```python
from build123d import *

# Parameters (mm, degrees)
SKETCH_1_W                  = 56
SKETCH_1_H                  = 90
SKETCH_1_R                  = 1.6
EXTRUDE_1_DEPTH             = 3
SKETCH_2_R                  = 18.5
SKETCH_2_R_2                = 1.6
CUT_EXTRUDE_1_DEPTH         = 54.08483776
FILLET_1_R                  = 2
CUT_EXTRUDE_2_DEPTH         = 54.08483776
FILLET_2_R                  = 2
HOLE_WIZARD_M3_1_AT_2_COUNT = 2
HOLE_WIZARD_M3_1_AT_2_PITCH = 63.694583757
HOLE_WIZARD_M3_1_AT_3_COUNT = 2
HOLE_WIZARD_M3_1_AT_3_PITCH = 63.694583757


with BuildPart() as part:
    # 草图1 → 凸台-拉伸1 (new body)
    with BuildSketch(Plane.XY):
        Rectangle(SKETCH_1_W, SKETCH_1_H)
        with Locations((10, 42)):
            Circle(SKETCH_1_R, mode=Mode.SUBTRACT)
        with Locations(Location((-10, 42, 0), (0, 0, 180))):
            Circle(SKETCH_1_R, mode=Mode.SUBTRACT)
    extrude(amount=EXTRUDE_1_DEPTH)

    # 草图2 → 切除-拉伸1 (cut, through all)
    with BuildSketch(Plane.XY.offset(3)):
        with Locations((0, -17)):
            Circle(SKETCH_2_R)
        with Locations((0, 18)):
            Circle(SKETCH_2_R_2)
        with Locations((24, -41)):
            Circle(SKETCH_2_R_2)
        with Locations(Location((-24, -41, 0), (0, 0, 180))):
            Circle(SKETCH_2_R_2)
    extrude(amount=-CUT_EXTRUDE_1_DEPTH, mode=Mode.SUBTRACT)

    # 圆角1
    fillet_1_edges = [part.edges().sort_by_distance(p)[0] for p in [
        (28, -45, 1.5),
        (-28, -45, 1.5),
        (-28, 45, 1.5),
        (28, 45, 1.5),
    ]]
    fillet(fillet_1_edges, radius=FILLET_1_R)

    # 草图3 → 切除-拉伸2 (cut, through all)
    with BuildSketch(Plane.XY.offset(3)):
        Polygon((-23.345028529, 37.432122744), (-4.29507275, 37.432122744), (-4.29507275, 6.166928146), (-23.345028529, -1.831144891), align=None)
        Polygon((4.29507275, 6.166928146), (23.345028529, -1.831144891), (23.345028529, 37.432122744), (4.29507275, 37.432122744), align=None)
        Polygon((-21.449213, -21.510239836), (-24.998316916, -30.185827186), (-17.308591765, -43.00203577), (-5.576831599, -43.00203577), (-16.421315786, -33.044827562), align=None)
        Polygon((21.449213, -21.510239836), (24.998316916, -30.185827186), (17.308591765, -43.00203577), (5.576831599, -43.00203577), (16.421315786, -33.044827562), align=None)
    extrude(amount=-CUT_EXTRUDE_2_DEPTH, mode=Mode.SUBTRACT)

    # 圆角2
    fillet_2_edges = [part.edges().sort_by_distance(p)[0] for p in [
        (-5.576831599, -43.00203577, 1.5),
        (-17.308591765, -43.00203577, 1.5),
        (-24.998316916, -30.185827186, 1.5),
        (-21.449213, -21.510239836, 1.5),
        (-16.421315786, -33.044827562, 1.5),
        (-23.345028529, -1.831144891, 1.5),
        (-23.345028529, 37.432122744, 1.5),
        (-4.29507275, 37.432122744, 1.5),
        (-4.29507275, 6.166928146, 1.5),
        (4.29507275, 6.166928146, 1.5),
        (4.29507275, 37.432122744, 1.5),
        (23.345028529, 37.432122744, 1.5),
        (23.345028529, -1.831144891, 1.5),
        (16.421315786, -33.044827562, 1.5),
        (21.449213, -21.510239836, 1.5),
        (24.998316916, -30.185827186, 1.5),
        (17.308591765, -43.00203577, 1.5),
        (5.576831599, -43.00203577, 1.5),
    ]]
    fillet(fillet_2_edges, radius=FILLET_2_R)

    # 草图5 → M3 十字槽半沉头木螺钉的锥形沉头孔1 (revolve, cut)
    with BuildSketch(Plane(origin=(0, 18, 0), x_dir=(0, 1, 0), z_dir=(1, 0, 0))):
        Polygon((0, 0), (0, 3), (1.8, 3), (1.8, 1.5), (3.3, 0), align=None)
    hole_wizard_m3_1 = revolve(axis=Axis((0, 18, -6.35), (0, 0, 1)), mode=Mode.SUBTRACT)

    # M3 十字槽半沉头木螺钉的锥形沉头孔1 at 2: M3 十字槽半沉头木螺钉的锥形沉头孔1 ×2
    with Locations(*[Vector(-0.3767981292019326, -0.9262954009547514, 0) * (i * HOLE_WIZARD_M3_1_AT_2_PITCH) for i in range(1, HOLE_WIZARD_M3_1_AT_2_COUNT)]):
        add(hole_wizard_m3_1, mode=Mode.SUBTRACT)

    # M3 十字槽半沉头木螺钉的锥形沉头孔1 at 3: M3 十字槽半沉头木螺钉的锥形沉头孔1 ×2
    with Locations(*[Vector(0.3767981292019329, -0.9262954009547514, 0) * (i * HOLE_WIZARD_M3_1_AT_3_PITCH) for i in range(1, HOLE_WIZARD_M3_1_AT_3_COUNT)]):
        add(hole_wizard_m3_1, mode=Mode.SUBTRACT)


solid = part.part
```
Model file for the job. Use its own axes, mm. A direction names the side the tool comes from. Give positions to 0.01 mm unless a question says otherwise; leave off trailing zeros. Loops run counter-clockwise (first coordinate to the right, second up) from the corner with the lowest first, then second, coordinate; pieces in that order, holes last. Notation, with made-up numbers: (20, 49.25) - (47, 49.25) arc R27 ccw to (47, 86.25) - close; hole circle Ø9 at (43.25, 62). An arc over 180 degrees is marked (long way). One line per item, written item: value. Start each with the question number.
1. Slice it at A-A (y = -17). List the corners of the cut face in (x, z), plus the area to 3 significant figures.
2. Slice it at B-B (x = 0). List the corners of the cut face in (y, z).
3. Slice it at C-C (y = 42). List the corners of the cut face in (x, z), plus the area to 3 significant figures.
4. Pull direction Y, two halves, no side cores. Call faces 3 (the flat face through (28, -1, 1)), 4 (the flat face through (21.233, -36.461, 1.521)), 5 (the cylindrical face through (-27.43, -44.4, 1.52)), 6 (the cylindrical face through (22.775, 36.831, 1.479)): pulls with the +Y half, pulls with the -Y half, needs draft (parallel to the pull), parting line crosses it, or undercut.
5. Pin check, flat tips, straight feed: pin 1 (5 mm diameter, centred on x = -10, y = 42, fed in from +Z); pin 2 (2.5 mm diameter, centred on x = 10, y = 42, fed in from -Z). Stop position of each tip, or through.
6. Probe L1, parallel to X at y = 10.5, z = 1; L2, parallel to X at y = 18, z = 2.45; L3, parallel to X at y = 2, z = 2.85. List the from-to ranges inside material, lowest first. Write a range as from..to.
7. Which spindle directions (+Z, -Z, +X, -X, +Y, -Y) get a long thin tool onto all of the face, cutting with end or side? Do faces 1 (the cylindrical face through (27.4, -44.43, 1.52)), 2 (the flat face through (14, 37.432, 2)). Say none if no direction does.
8. Slice it at D-D (y = 18). List the corners of the cut face in (x, z), plus the area to 3 significant figures.
Solution:
1. outline: (-28, 0) - (-18.5, 0) - (-18.5, 3) - (-28, 3) - close; (18.5, 0) - (28, 0) - (28, 3) - (18.5, 3) - close
1. area: 57.0 mm^2
2. outline: (-45, 0) - (-35.5, 0) - (-35.5, 3) - (-45, 3) - close; (1.5, 0) - (14.7, 0) - (16.2, 1.5) - (16.2, 3) - (1.5, 3) - close; (19.8, 1.5) - (21.3, 0) - (45, 0) - (45, 3) - (19.8, 3) - close
3. outline: (-28, 0) - (-11.6, 0) - (-11.6, 3) - (-28, 3) - close; (-8.4, 0) - (8.4, 0) - (8.4, 3) - (-8.4, 3) - close; (11.6, 0) - (28, 0) - (28, 3) - (11.6, 3) - close
3. area: 149 mm^2
4. face 3: needs draft
4. face 4: undercut
4. face 5: pulls with the -Y half
4. face 6: undercut
5. pin 1: stops at z = 3
5. pin 2: passes through
6. L1: x = -28..-23.35, -4.3..4.3, 23.35..28
6. L2: x = -28..-23.35, -4.3..-1.8, 1.8..4.3, 23.35..28
6. L3: x = -28..-23.35, -14.22..14.22, 23.35..28
7. face 1: +Z, -Z, +X, -Y
7. face 2: +Z, -Z
8. outline: (-28, 0) - (-23.35, 0) - (-23.35, 3) - (-28, 3) - close; (-4.3, 0) - (-3.3, 0) - (-1.8, 1.5) - (-1.8, 3) - (-4.3, 3) - close; (1.8, 1.5) - (3.3, 0) - (4.3, 0) - (4.3, 3) - (1.8, 3) - close; (23.35, 0) - (28, 0) - (28, 3) - (23.35, 3) - close
8. area: 40.7 mm^2
